from build123d import *

# Parameters (mm, degrees)
F0_W      = 15.7988
F0_H      = 27.686
F1_DEPTH  = 10.033
F2_R      = 1.6891
F3_DEPTH  = 10.033
F4_W      = 0.8128
F4_H      = 3.175
F5_DEPTH  = 3.81
F6_W      = 0.8128
F6_H      = 6.35
F7_DEPTH  = 15.748
F8_R      = 1.27
F9_SIZE   = 1.27
F10_W     = 0.8128
F10_H     = 3.175
F11_DEPTH = 3.175
F13_DEPTH = 6.35
F14_W     = 1.1494727835
F14_H     = 6.35
F15_DEPTH = 2.54
F17_DEPTH = 6.35
F18_W     = 0.8128
F18_H     = 6.35
F19_DEPTH = 9.906
F20_R     = 1.27
F21_SIZE  = 1.27
F22_W     = 0.8128
F22_H     = 2.2987
F23_DEPTH = 1.27
F25_DEPTH = 4.5974
F26_W     = 1.9280109734
F26_H     = 4.5974
F27_DEPTH = 12.7
F28_W     = 4.6482
F28_H     = 4.5974
F29_DEPTH = 5.715
F30_R     = 2.032
F31_R     = 1.27


with BuildPart() as f1:
    # F0 (on Top) → F1 (new body)
    with BuildSketch(Plane.XY):
        Rectangle(F0_W, F0_H)
    extrude(amount=F1_DEPTH)

    # F2 (on face) → F3 (cut, through all)
    with BuildSketch(Plane.XY.offset(10.033)):
        with Locations((5.0419, 10.9855)):
            Circle(F2_R)
        with Locations((-5.0419, -10.9855)):
            Circle(F2_R)
    extrude(amount=-F3_DEPTH, mode=Mode.SUBTRACT)

    # F4 (on face) → F5 (join)
    with BuildSketch(Plane.YZ.offset(7.8994)):
        with Locations((3.1242, 6.604)):
            Rectangle(F4_W, F4_H)
        with Locations((3.1242, 3.429)):
            Rectangle(F4_W, F4_H)
    extrude(amount=F5_DEPTH)

    # F6 (on face) → F7 (join)
    with BuildSketch(Plane.XZ.offset(-2.7178)):
        with Locations((11.303, 5.0165)):
            Rectangle(F6_W, F6_H)
    extrude(amount=F7_DEPTH)

    # F8
    f8_edges = [f1.edges().sort_by_distance(p)[0] for p in [
        (11.7094, 3.5306, 5.0165),
        (10.8966, 2.7178, 5.0165),
    ]]
    fillet(f8_edges, radius=F8_R)

    # F9
    f9_edges = [f1.edges().sort_by_distance(p)[0] for p in [
        (11.303, -13.0302, 8.1915),
        (11.303, -13.0302, 1.8415),
    ]]
    chamfer(f9_edges, length=F9_SIZE)

    # F10 (on face) → F11 (join)
    with BuildSketch(Plane.XZ.offset(13.843)):
        with Locations((4.699, 6.604)):
            Rectangle(F10_W, F10_H)
        with Locations((4.699, 3.429)):
            Rectangle(F10_W, F10_H)
    extrude(amount=F11_DEPTH)

    # F12 (on face) → F13 (join, through all)
    with BuildSketch(Plane.XY.offset(8.1915)):
        Polygon((4.2926, -17.8308), (5.1054, -17.018), (4.2926, -17.018), align=None)
    extrude(amount=-F13_DEPTH)

    # F14 (on face) → F15 (join)
    with BuildSketch(Plane(origin=(11.0617, -11.0617, 0), x_dir=(0.7071067812, 0.7071067812, 0), z_dir=(0.7071067812, -0.7071067812, 0))):
        with Locations((-8.9982166333, 5.0165)):
            Rectangle(F14_W, F14_H)
    extrude(amount=F15_DEPTH)

    # F16 (on face) → F17 (join, through all)
    with BuildSketch(Plane.XY.offset(8.1915)):
        Polygon((6.9014512242, -19.6268512242), (6.9014512242, -18.8140512242), (6.0886512242, -19.6268512242), align=None)
    extrude(amount=-F17_DEPTH)

    # F18 (on face) → F19 (join)
    with BuildSketch(Plane.XZ.offset(19.6268512242)):
        with Locations((6.4950512242, 5.0165)):
            Rectangle(F18_W, F18_H)
    extrude(amount=F19_DEPTH)

    # F20
    f20_edges = [f1.edges().sort_by_distance(p)[0] for p in [
        (4.2926, -17.8308, 5.0165),
        (5.1054, -17.018, 5.0165),
        (6.901451, -18.814051, 5.0165),
        (6.088651, -19.626851, 5.0165),
    ]]
    fillet(f20_edges, radius=F20_R)

    # F21
    f21_edges = [f1.edges().sort_by_distance(p)[0] for p in [
        (6.495051, -29.532851, 1.8415),
        (6.495051, -29.532851, 8.1915),
    ]]
    chamfer(f21_edges, length=F21_SIZE)

    # F22 (on face) → F23 (join)
    with BuildSketch(Plane(origin=(-7.8994, 0, 0), x_dir=(0, -1, 0), z_dir=(-1, 0, 0))):
        with Locations((-1.905, 3.86715)):
            Rectangle(F22_W, F22_H)
        with Locations((-1.905, 6.16585)):
            Rectangle(F22_W, F22_H)
    extrude(amount=F23_DEPTH)

    # F24 (on face) → F25 (join, through all)
    with BuildSketch(Plane.XY.offset(7.3152)):
        Polygon((-9.1694, 1.4986), (-9.1694, 1.5813095502), (-11.0637601465, 1.4986), align=None)
    extrude(amount=-F25_DEPTH)

    # F26 (on face) → F27 (join)
    with BuildSketch(Plane(origin=(-0.0863562718, 1.9778838039, 0), x_dir=(-0.9990482216, -0.0436193874, 0), z_dir=(-0.0436193874, 0.9990482216, 0))):
        with Locations((10.0238563977, 5.0165)):
            Rectangle(F26_W, F26_H)
    extrude(amount=F27_DEPTH)

    # F28 (on face) → F29 (join)
    with BuildSketch(Plane(origin=(-10.9774038747, -0.4792838039, 0), x_dir=(0.0436193874, -0.9990482216, 0), z_dir=(-0.9990482216, -0.0436193874, 0))):
        with Locations((-12.3556681044, 5.0165)):
            Rectangle(F28_W, F28_H)
    extrude(amount=F29_DEPTH)

    # F30
    f30_edges = [f1.edges().sort_by_distance(p)[0] for p in [
        (-17.124535, 9.293452, 5.0165),
        (-17.327287, 13.937228, 5.0165),
    ]]
    fillet(f30_edges, radius=F30_R)

    # F31
    f31_edges = [f1.edges().sort_by_distance(p)[0] for p in [
        (-16.706734, 13.368596, 7.3152),
        (-16.555903, 9.914005, 7.3152),
        (-17.225911, 11.61534, 7.3152),
        (-17.225911, 11.61534, 2.7178),
        (-16.555903, 9.914005, 2.7178),
        (-16.706734, 13.368596, 2.7178),
    ]]
    fillet(f31_edges, radius=F31_R)


solid = f1.part
Read the model definition and answer for the solid it produces. Units are mm, in the model's axes. A direction names the side the tool comes from. Round coordinates to 2 decimals unless told otherwise and drop trailing zeros. Write each loop counter-clockwise with the first axis right and the second up, starting at its lowest first coordinate (ties: lowest second). Pieces come first, ordered by that corner, then holes.
Q1. A tool of negligible diameter and unlimited length cuts with its end or side. For faces 1 (the face through (11.297, -12.404, 2.485)), 2 (the face through (11.3, -2.9, 1.842)), 3 (the face through (11.297, -12.386, 7.565)), 4 (the face through (9, 3.531, 5)), from which of +Z, -Z, +X, -X, +Y, -Y can it reach the whole face along a straight path? Write none if from no direction.
Values:
face 1: -Z, +X, -Y
face 2: -Z, +X, +Y, -Y
face 3: +Z, +X, -Y
face 4: +Z, -Z, +X, +Y
Q2. Find section D-D on y = -22. Determine the outline of the cut face in (x, z), and give its area (3 significant figures).
Values:
outline: (6.09, 1.84) - (6.9, 1.84) - (6.9, 8.19) - (6.09, 8.19) - close
area: 5.16 mm2
Q3. Find section A-A on y = -2.5. Determine the outline of the cut face in (x, z).
Values:
outline: (-7.9, 0) - (7.9, 0) - (7.9, 10.03) - (-7.9, 10.03) - close; (10.9, 1.84) - (11.71, 1.84) - (11.71, 8.19) - (10.9, 8.19) - close
Q4. Straight lines are drawn through the part: line 1 (X direction, y = -1.5, z = 7.5); line 2 (X direction, y = -15.5, z = 3.5); line 3 (Y direction, x = -8, z = 4.5). For each, find the intervals that lie inside material, in ascending order.
Values:
line 1: x = -7.9 to 7.9, 10.9 to 11.71
line 2: x = 4.29 to 5.11
line 3: y = 1.5 to 2.31
Q5. Flat-ended cylindrical pins translate along their axes: P1, Ø4, axis at x = -13, y = 9, coming from the -Z side; P2, Ø4, axis at y = -18, z = 5, coming from the -X side; P3, Ø1.9, axis at x = 8.5, z = 5.5, coming from the -Y side. Find the tip coordinate at first contact, or state that the pin passes through.
Values:
P1: stops at z = 2.72
P2: stops at x = 4.29
P3: stops at y = -13.84
Q6. Find section C-C on y = 7. Determine the outline of the cut face in (x, z), and give its area (3 significant figures).
Values:
outline: (-11.3, 2.72) - (-9.37, 2.72) - (-9.37, 7.32) - (-11.3, 7.32) - close; (-7.9, 0) - (7.9, 0) - (7.9, 10.03) - (-7.9, 10.03) - close
area: 167 mm2
Q7. Find section B-B on z = 8.75. Determine the outline of the cut face in (x, y), and give its area (3 significant figures).
Values:
outline: (-7.9, -13.84) - (7.9, -13.84) - (7.9, 13.84) - (-7.9, 13.84) - close; hole circle Ø3.38 at (-5.04, -10.99); hole circle Ø3.38 at (5.04, 10.99)
area: 419 mm2
Q8. The mould has two halves that part along X. Classify faces 5 (the face through (-16.844, 11.628, 3.08)), 6 (the face through (-7.899, 0, 5)), 7 (the face through (0, 13.843, 5)): released by +X, released by -X, zero draft, split by the parting line, or undercut.
Values:
face 5: released by -X
face 6: undercut
face 7: zero draft
